```python
from build123d import *

# Parameters (mm, degrees)
BASE_FLANGE1_DEPTH = 32
CUT_EXTRUDE1_REACH = 130.658
SKETCH7_R          = 1.5
CUT_EXTRUDE2_REACH = 131.808
SKETCH8_R          = 5.5
FILLET1_R          = 3


# Sheet-metal steps are written as plain solids
with BuildPart() as part:
    # Sketch2 → Base-Flange1 (new body)
    with BuildSketch(Plane(origin=(0, 0, 0), x_dir=(1, 0, 0), z_dir=(0, 1, 0))):
        with BuildLine():
            Line((-115, 48), (-76, 48))
            ThreePointArc((-76, 48), (-71.757359313, 46.242640687), (-70, 42))
            Line((-70, 42), (-70, 3))
            ThreePointArc((-70, 3), (-69.121320344, 0.878679656), (-67, 0))
            Line((-67, 0), (0, 0))
            Line((0, 0), (0, -3))
            Line((0, -3), (-67, -3))
            ThreePointArc((-67, -3), (-71.242640687, -1.242640687), (-73, 3))
            Line((-73, 3), (-73, 42))
            ThreePointArc((-73, 42), (-73.878679656, 44.121320344), (-76, 45))
            Line((-76, 45), (-115, 45))
            Line((-115, 45), (-115, 48))
        make_face()
    extrude(amount=BASE_FLANGE1_DEPTH)

    # Sketch7 → Cut-Extrude1 (cut, up to next)
    with BuildSketch(Plane.XY.offset(-45), mode=Mode.PRIVATE) as cut_extrude1_sk1:
        with Locations((-103, 23)):
            Circle(SKETCH7_R)
    cut_extrude1_tool1 = extrude(cut_extrude1_sk1.sketch, amount=-CUT_EXTRUDE1_REACH, mode=Mode.PRIVATE) & part.part
    # Sketch7 → Cut-Extrude1 (cut, up to next)
    with BuildSketch(Plane.XY.offset(-45), mode=Mode.PRIVATE) as cut_extrude1_sk2:
        with Locations((-103, 9)):
            Circle(SKETCH7_R)
    cut_extrude1_tool2 = extrude(cut_extrude1_sk2.sketch, amount=-CUT_EXTRUDE1_REACH, mode=Mode.PRIVATE) & part.part
    add(cut_extrude1_tool1.solids().sort_by_distance((-103, 23, -45))[0], mode=Mode.SUBTRACT)
    add(cut_extrude1_tool2.solids().sort_by_distance((-103, 9, -45))[0], mode=Mode.SUBTRACT)

    # Sketch8 → Cut-Extrude2 (cut, up to next)
    with BuildSketch(Plane.XY.offset(3), mode=Mode.PRIVATE) as cut_extrude2_sk1:
        with Locations((-15, 16)):
            Circle(SKETCH8_R)
    cut_extrude2_tool1 = extrude(cut_extrude2_sk1.sketch, amount=-CUT_EXTRUDE2_REACH, mode=Mode.PRIVATE) & part.part
    add(cut_extrude2_tool1.solids().sort_by_distance((-15, 16, 3))[0], mode=Mode.SUBTRACT)

    # Fillet1
    fillet1_edges = [part.edges().sort_by_distance(p)[0] for p in [
        (-115, 0, -46.5),
        (0, 0, 1.5),
        (-115, 32, -46.5),
        (0, 32, 1.5),
    ]]
    fillet(fillet1_edges, radius=FILLET1_R)


solid = part.part
```
Build history of the part. All positions in model axes, mm. A direction names the side the tool comes from. Coordinates: 2 decimals unless noted, no trailing zeros. Write each loop counter-clockwise with the first axis right and the second up, starting at its lowest first coordinate (ties: lowest second). Pieces come first, ordered by that corner, then holes.
1. Band-saw the part on D-D, the plane y = 16. Give the cut face in (x, z).
Answer block:
outline: (-115, -48) - (-76, -48) arc R6 ccw to (-70, -42) - (-70, -3) arc R3 cw to (-67, 0) - (-20.5, 0) - (-20.5, 3) - (-67, 3) arc R6 ccw to (-73, -3) - (-73, -42) arc R3 cw to (-76, -45) - (-115, -45) - close; (-9.5, 0) - (0, 0) - (0, 3) - (-9.5, 3) - close
2. Band-saw the part on B-B, the plane x = -103. Give the cut face in (y, z), and give its area (3 significant figures).
Answer block:
outline: (0, -48) - (7.5, -48) - (7.5, -45) - (0, -45) - close; (10.5, -48) - (21.5, -48) - (21.5, -45) - (10.5, -45) - close; (24.5, -48) - (32, -48) - (32, -45) - (24.5, -45) - close
area: 78.0 mm2
3. Drill centre lines: probe 1 along Y at (x, z) = (-103, -47.1); probe 2 along Y at (x, z) = (-15, 2.25); probe 3 along Z at (x, y) = (-24, 14). Where is each one in solid material? Low to high.
Answer block:
probe 1: y = 0 to 7.5, 10.5 to 21.5, 24.5 to 32
probe 2: y = 0 to 10.5, 21.5 to 32
probe 3: z = 0 to 3
4. Band-saw the part on C-C, the plane x = -15. Give the cut face in (y, z), and give its area (3 significant figures).
Answer block:
outline: (0, 0) - (10.5, 0) - (10.5, 3) - (0, 3) - close; (21.5, 0) - (32, 0) - (32, 3) - (21.5, 3) - close
area: 63.0 mm2
5. Drop flat-ended pins along their axis: pin 1 (1 mm diameter, centred on x = -54.5, y = 11.5, fed in from -Z); pin 2 (9.5 mm diameter, centred on y = 12.5, z = -24.5, fed in from +X); pin 3 (16 mm diameter, centred on y = 12, z = -27, fed in from -X). Give the stop position or say it passes through.
Answer block:
pin 1: stops at z = 0
pin 2: stops at x = -70
pin 3: stops at x = -73
6. Band-saw the part on A-A, the plane y = 9. Give the cut face in (x, z).
Answer block:
outline: (-115, -48) - (-104.5, -48) - (-104.5, -45) - (-115, -45) - close; (-101.5, -48) - (-76, -48) arc R6 ccw to (-70, -42) - (-70, -3) arc R3 cw to (-67, 0) - (0, 0) - (0, 3) - (-67, 3) arc R6 ccw to (-73, -3) - (-73, -42) arc R3 cw to (-76, -45) - (-101.5, -45) - close
7. 3-axis set-ups, long thin cutter, end or side, ignore diameter. For faces 4 (the cylindrical face through (-0.9, 0.86, 1.52)), 5 (the flat face through (-95, 16, -45)), 6 (the flat face through (-34, 16, 0)): which of +Z, -Z, +X, -X, +Y, -Y reach the whole face in a straight line?
Answer block:
face 4: +Z, -Z, +X, -Y
face 5: +Z, -X, +Y, -Y
face 6: -Z, +X, +Y, -Y
8. Pull direction X, two halves, no side cores. Call faces 1 (the cylindrical face through (-16.19, 10.63, 1.52)), 2 (the flat face through (-73, 16, -22)), 3 (the cylindrical face through (-69.14, 15.78, -0.9)): released by +X, released by -X, zero draft, split by the parting line, or undercut.
Answer block:
face 1: undercut
face 2: released by -X
face 3: released by +X
